```python
from build123d import *

# Parameters (mm, degrees)
F0_R     = 6
F0_W     = 6
F0_H     = 6
F1_DEPTH = 6
F0_R_2   = 17.2321789882
F2_DEPTH = 5
F3_DEPTH = 5
F0_R_3   = 20
F4_DEPTH = 15
F5_R     = 17.4069138817
F5_R_2   = 6
F6_DEPTH = 5


with BuildPart() as f1:
    # F0 (on Front) → F1 (new body)
    with BuildSketch(Plane.XZ):
        Circle(F0_R)
        Rectangle(F0_W, F0_H, mode=Mode.SUBTRACT)
    extrude(amount=F1_DEPTH)

    # F0 (on Front) → F2 (join)
    with BuildSketch(Plane.XZ):
        Circle(F0_R_2)
        Circle(F0_R, mode=Mode.SUBTRACT)
    extrude(amount=F2_DEPTH)

    # F0 (on Front) → F3 (join)
    with BuildSketch(Plane.XZ):
        Circle(F0_R)
        Rectangle(F0_W, F0_H, mode=Mode.SUBTRACT)
    extrude(amount=F3_DEPTH)

    # F0 (on Front) → F4 (join)
    with BuildSketch(Plane.XZ):
        Circle(F0_R_3)
        Circle(F0_R_2, mode=Mode.SUBTRACT)
        Circle(F0_R_2)
        Circle(F0_R, mode=Mode.SUBTRACT)
    extrude(amount=F4_DEPTH)

    # F5 (on face) → F6 (cut)
    with BuildSketch(Plane.XZ.offset(15)):
        Circle(F5_R)
        Circle(F5_R_2, mode=Mode.SUBTRACT)
    extrude(amount=-F6_DEPTH, mode=Mode.SUBTRACT)


solid = f1.part
```
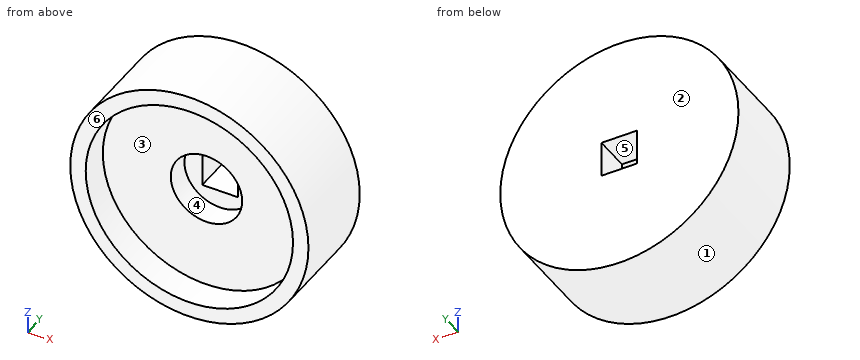
Geometry check sheet. Reference: the model listing, model coordinates, mm. Face numbers are marked on the shaded views. A direction names the side the tool comes from. Round coordinates to 2 decimals unless told otherwise and drop trailing zeros. Order: outer loops, then holes, each group sorted by start corner. A loop starts at its lowest first (then second) coordinate and runs counter-clockwise, first axis right, second up. Notation, with made-up numbers: (56, 8) - (60, 8) arc R9 cw to (60, 25) - close; hole circle Ø6 at (61.5, 66.5). An arc over 180 degrees is marked (long way). Use a Markdown table: item, result. Add a question column.
(1) Material ranges on line 1 along Z through (x, y) = (0.5, -13.5); line 2 along Z through (x, y) = (0, -7.5); line 3 along Y through (x, z) = (13, -2.5), recorded low to high. Write a range as [from, to].
(2) Sectioned sample at B-B, the plane z = 0. Enter the section's corners in (x, y).
(3) Sectioned sample at C-C, the plane y = -5.5. Enter the section's corners in (x, z).
(4) Sectioned sample at A-A, the plane x = 0. Enter the section's corners in (y, z), and give its area (3 significant figures).
(5) Sectioned sample at D-D, the plane x = -4.5. Enter the section's corners in (y, z).
(6) Release check for a two-part mould opening along Z. For the marked faces 1, 2 and 3 record: pulls with the +Z half, pulls with the -Z half, needs draft (parallel to the pull), parting line crosses it, or undercut.
(7) Tool access check on the marked faces 4, 5 and 6. Record the directions out of +Z, -Z, +X, -X, +Y, -Y that give a thin tool (end or side, any length) a straight path to the whole face; none if there is none.
(8) Depth check by flat-ended pin: pin 1 (3 mm diameter, centred on x = -1, y = -3, fed in from -Z); pin 2 (7 mm diameter, centred on x = 0, z = 0, fed in from -Y); pin 3 (2 mm diameter, centred on x = -12.5, y = -7.5, fed in from +Z); pin 4 (8 mm diameter, centred on y = -9, z = -3, fed in from -X). Enter the tip coordinate at first touch or a pass-through.
Answers below:
| question | item | result |
|---|---|---|
| 1 | line 1 | [-19.99, -17.4], [17.4, 19.99] |
| 1 | line 2 | [-20, -6], [6, 20] |
| 1 | line 3 | [-10, 0] |
| 2 | outline | (-20, -15) - (-17.41, -15) - (-17.41, -10) - (-6, -10) - (-6, -6) - (-3, -6) - (-3, 0) - (-20, 0) - close; (3, -6) - (6, -6) - (6, -10) - (17.41, -10) - (17.41, -15) - (20, -15) - (20, 0) - (3, 0) - close |
| 3 | outline | circle Ø40 at (0, 0); hole (-3, -3) - (3, -3) - (3, 3) - (-3, 3) - close |
| 4 | outline | (-15, -20) - (0, -20) - (0, -3) - (-6, -3) - (-6, -6) - (-10, -6) - (-10, -17.41) - (-15, -17.41) - close; (-15, 17.41) - (-10, 17.41) - (-10, 6) - (-6, 6) - (-6, 3) - (0, 3) - (0, 20) - (-15, 20) - close |
| 4 | area | 342 mm² |
| 5 | outline | (-15, -19.49) - (0, -19.49) - (0, 19.49) - (-15, 19.49) - (-15, 16.82) - (-10, 16.82) - (-10, 3.97) - (-6, 3.97) - (-6, -3.97) - (-10, -3.97) - (-10, -16.82) - (-15, -16.82) - close |
| 6 | face 1 | parting line crosses it |
| 6 | face 2 | needs draft |
| 6 | face 3 | undercut |
| 7 | face 4 | -Y |
| 7 | face 5 | +Y, -Y |
| 7 | face 6 | +Z, -Z, +X, -X, -Y |
| 8 | pin 1 | z = -20 |
| 8 | pin 2 | y = -6 |
| 8 | pin 3 | z = 16.36 |
| 8 | pin 4 | x = -20 |
